from build123d import *

# Parameters (mm, degrees)
SKETCH1_W           = 1500
SKETCH1_H           = 600
BOSS_EXTRUDE1_DEPTH = 300
BOSS_EXTRUDE2_DEPTH = 30


with BuildPart() as part:
    # Sketch1 → Boss-Extrude1 (new body)
    with BuildSketch(Plane(origin=(0, 0, 0), x_dir=(1, 0, 0), z_dir=(0, 1, 0))):
        Rectangle(SKETCH1_W, SKETCH1_H)
    extrude(amount=BOSS_EXTRUDE1_DEPTH)

    # Sketch2 → Boss-Extrude2 (add)
    with BuildSketch(Plane(origin=(0, 300, 0), x_dir=(1, 0, 0), z_dir=(0, 1, 0))):
        with BuildLine():
            Line((-75, -300), (75, -300))
            ThreePointArc((75, -300), (0, -525), (-75, -300))
        make_face()
        with BuildLine():
            Line((-75, 300), (75, 300))
            ThreePointArc((75, 300), (0, 525), (-75, 300))
        make_face()
        with BuildLine():
            Line((625, -300), (475, -300))
            ThreePointArc((475, -300), (550, -525), (625, -300))
        make_face()
        with BuildLine():
            Line((625, 300), (475, 300))
            ThreePointArc((475, 300), (550, 525), (625, 300))
        make_face()
        with BuildLine():
            Line((-475, -300), (-625, -300))
            ThreePointArc((-625, -300), (-550, -525), (-475, -300))
        make_face()
        with BuildLine():
            Line((-475, 300), (-625, 300))
            ThreePointArc((-625, 300), (-550, 525), (-475, 300))
        make_face()
    extrude(amount=-BOSS_EXTRUDE2_DEPTH)


solid = part.part
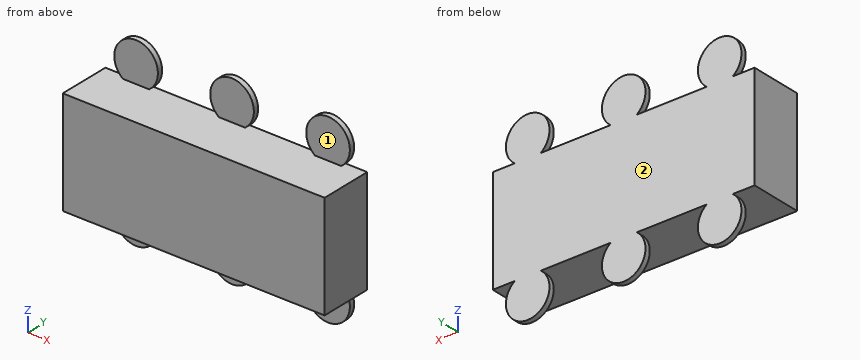
Verification items for the finished model (mm, model axes). Face numbers are marked on the shaded views. A direction names the side the tool comes from. Give positions to 0.01 mm unless a question says otherwise; leave off trailing zeros. Loops run counter-clockwise (first coordinate to the right, second up) from the corner with the lowest first, then second, coordinate; pieces in that order, holes last. Notation, with made-up numbers: (-25.75, 15.25) - (-13.75, 15.25) arc R7 cw to (-13.75, 19.25) - close; hole circle Ø7 at (-15.75, 8). An arc over 180 degrees is marked (long way). Write each question's results on one line, items separated by ' | '.
1) Tool access check on the marked faces 1 and 2. Record the directions out of +Z, -Z, +X, -X, +Y, -Y that give a thin tool (end or side, any length) a straight path to the whole face; none if there is none.
Solution:
face 1: +Z, +X, -X, -Y | face 2: +Z, -Z, +X, -X, +Y
2) Material ranges on L1, parallel to X at y = 280, z = -379; L2, parallel to X at y = 273, z = -433; L3, parallel to Z at x = 157, y = 98.5, recorded low to high. Write a range as from..to.
Solution:
L1: -673.22..-426.78, -123.22..123.22, 426.78..673.22 | L2: -670.57..-429.43, -120.57..120.57, 429.43..670.57 | L3: -300..300
3) Sectioned sample at D-D on x = -645.5. Record the boundary of the cut face in (y, z).
Solution:
outline: (0, -300) - (300, -300) - (300, 300) - (0, 300) - close; (270, -480.65) - (300, -480.65) - (300, -319.35) - (270, -319.35) - close; (270, 319.35) - (300, 319.35) - (300, 480.65) - (270, 480.65) - close
4) Depth check by flat-ended pin: P1, Ø10, axis at x = 267.5, y = 83.5, coming from the +Z side; P2, Ø1.5, axis at x = -377.5, y = 47, coming from the -Z side. Enter the tip coordinate at first touch or a pass-through.
Solution:
P1: z = 300 | P2: z = -300
5) Sectioned sample at A-A on z = 400. Record the boundary of the cut face in (x, y), plus the area to 3 significant figures.
Solution:
outline: (-675, 270) - (-425, 270) - (-425, 300) - (-675, 300) - close; (-125, 270) - (125, 270) - (125, 300) - (-125, 300) - close; (425, 270) - (675, 270) - (675, 300) - (425, 300) - close | area: 22,500 mm2
6) Sectioned sample at C-C on y = 123.5. Record the boundary of the cut face in (x, z).
Solution:
outline: (-750, -300) - (750, -300) - (750, 300) - (-750, 300) - close
7) Sectioned sample at B-B on x = 550. Record the boundary of the cut face in (y, z).
Solution:
outline: (0, -300) - (270, -300) - (270, -525) - (300, -525) - (300, 525) - (270, 525) - (270, 300) - (0, 300) - close
